from build123d import *

# Parameters (mm, degrees)
SKETCH002_R       = 5.05
PAD001_DEPTH      = 2
POCKET_DEPTH      = 2
POCKET_DEPTH_BACK = -2


with BuildPart() as part:
    # Sketch002 → Pad001 (new body)
    with BuildSketch(Plane.XY):
        with Locations((-1, 0)):
            Circle(SKETCH002_R)
    extrude(amount=PAD001_DEPTH)

    # Sketch → Pocket (cut, two sides)
    with BuildSketch(Plane.XY) as pocket_sk:
        with BuildLine():
            ThreePointArc((1.5, 2), (0, 2.5), (-1.5, 2))
            Line((-1.5, -2), (-1.5, 2))
            ThreePointArc((-1.5, -2), (0, -2.5), (1.5, -2))
            Line((1.5, 2), (1.5, -2))
        make_face()
    extrude(amount=-POCKET_DEPTH, mode=Mode.SUBTRACT)
    extrude(pocket_sk.sketch, amount=-POCKET_DEPTH_BACK, mode=Mode.SUBTRACT)


solid = part.part
Verification items for the finished model (mm, model axes). A direction names the side the tool comes from. Give positions to 0.01 mm unless a question says otherwise; leave off trailing zeros. Write each loop counter-clockwise with the first axis right and the second up, starting at its lowest first coordinate (ties: lowest second). Pieces come first, ordered by that corner, then holes. Notation, with made-up numbers: M 27,-40 L 53,-40 A27 ccw 53,-6 Z; hole C 63,23 d1. An arc over 180 degrees is marked long. Put each result on its own line as item: value. Start each with the question number.
1. Section check A-A (x = 0). Record the cut outline in (y, z).
2. Section check B-B (y = 0). Record the cut outline in (x, z).
3. Section check C-C (z = 0.2). Record the cut outline in (x, y).
4. Set-up check for faces 4 (the face through (-2, 0, 2)), 5 (the face through (0, 2.5, 1)): record each of +Z, -Z, +X, -X, +Y, -Y from which the full face is reachable in a straight line by a thin tool's end or side.
5. Section check D-D (y = 3.5). Record the cut outline in (x, z).
6. Draft check along X on faces 1 (the face through (-2, 0, 0)), 2 (the face through (3.817, 1.517, 0.986)), 3 (the face through (1.5, 0, 1)). Enter one of: +X half, -X half, draft (parallel to the pull), parting line (faces both ways), or undercut.
7. Scan lines: line 1 along X through (y, z) = (1.75, 1.6); line 2 along Y through (x, z) = (0.75, 1.1); line 3 along X through (y, z) = (-1.25, 0.7). Record each from-to range of solid material in increasing order. Write a range as [from, to].
Answer list:
1. outline: M -4.95,0 L -2.5,0 L -2.5,2 L -4.95,2 Z; M 2.5,0 L 4.95,0 L 4.95,2 L 2.5,2 Z
2. outline: M -6.05,0 L -1.5,0 L -1.5,2 L -6.05,2 Z; M 1.5,0 L 4.05,0 L 4.05,2 L 1.5,2 Z
3. outline: C -1,0 d10.1; hole M -1.5,-2 A2.5 ccw 1.5,-2 L 1.5,2 A2.5 ccw -1.5,2 Z
4. face 4: +Z, +X, -X, +Y, -Y
4. face 5: +Z, -Z
5. outline: M -4.64,0 L 2.64,0 L 2.64,2 L -4.64,2 Z
6. face 1: draft
6. face 2: parting line
6. face 3: undercut
7. line 1: [-5.74, -1.5], [1.5, 3.74]
7. line 2: [-4.74, -2.38], [2.38, 4.74]
7. line 3: [-5.89, -1.5], [1.5, 3.89]
